Autodesk Inventor part; units mm, degrees
ref_plane "YZ Plane" through (0, 0, 0) normal (1, 0, 0) x (0, 1, 0)
ref_plane "XZ Plane" through (0, 0, 0) normal (0, 1, 0) x (-1, 0, 0)
ref_plane "XY Plane" through (0, 0, 0) normal (0, 0, 1) x (1, 0, 0)
sketch "Boceto1" plane through (0, 0, 0) normal (0, 1, 0) x (-1, 0, 0)
  line L0 (-50, 50) -> (50, 50)
  line L1 (50, 50) -> (50, -50)
  line L2 (50, -50) -> (-50, -50)
  line L3 (-50, -50) -> (-50, 50)
  line L4 (-50, 50) -> (50, -50) construction
  line L5 (50, 50) -> (-50, -50) construction
  point P0 (0, 0)
  dimension "d0" = 100
  dimension "d1" = 100
extrude "Extrusión1" add sketch "Boceto1" along normal blind 10
sketch "Boceto3" plane through (0, 10, 0) normal (0, 1, 0) x (1, 0, 0)
  point P0 (0, 0)
sketch "Boceto4" plane through (0, 10, 0) normal (0, 1, 0) x (1, 0, 0)
  circle A0 centre (0, 0) radius 45
  dimension "d5" = 90
extrude "Extrusión2" add sketch "Boceto4" along normal blind 20.06
sketch "Boceto5" plane through (0, 30.06, 0) normal (0, 1, 0) x (1, 0, 0)
  circle A0 centre (0, 0) radius 50
extrude "Extrusión3" add sketch "Boceto5" along normal blind 10
sketch "Boceto6" plane through (0, 40.06, 0) normal (0, 1, 0) x (1, 0, 0)
  circle A0 centre (0, 0) radius 15.325
  dimension "d10" = 30.65
hole "Agujero1" at (0, 40.06, 0) direction (0, -1, 0) diameter 30.65 end through all
properties part number "base de las bobinas"
Geometry: final body of the model. Coordinates: model frame, mm. A direction names the side the tool comes from. Coordinates: 2 decimals unless noted, no trailing zeros. Loops run counter-clockwise (first coordinate to the right, second up) from the corner with the lowest first, then second, coordinate; pieces in that order, holes last. Notation, with made-up numbers: M 31,9 L 35,9 A35 cw 35,42 Z; hole C 38,-22 d5. An arc over 180 degrees is marked long. One line per item, written item: value. Start each with the question number.
1) Cut plane A-A (z = 0). Return loops of the section in (x, y) (3 decimals), then the cut area to 3 significant figures.
2) Cut plane C-C (y = 35.5). Return loops of the section in (x, z) (3 decimals), then the cut area to 3 significant figures.
3) Material intervals for L1, parallel to Z at x = 0, y = 11 (3 decimals); L2, parallel to Y at x = 46.5, z = -11, sorted ascending. Write a range as from..to.
4) Pin query (flat end, axial travel): P1, Ø1.5, axis at x = -20, y = 35, coming from the +Z side; P2, Ø12, axis at y = 15, z = -18, coming from the -X side; P3, Ø6, axis at x = -37.5, y = 33.5, coming from the -Z side; P4, Ø4, axis at y = 22.5, z = 10.5, coming from the +X side. Return the tip coordinate at first contact, or that it passes through.
5) Draft query along Y for faces 1 (the flat face through (12, 0, 12)), 2 (the cylindrical face through (-12.92, 19.75, 8.24)), 3 (the cylindrical face through (20.765, 19.89, -39.923)). Return one class per face: released by +Y, released by -Y, zero draft, split by the parting line, or undercut.
6) Cut plane D-D (x = -22.5). Return loops of the section in (y, z), then the cut area to 3 significant figures.
7) Cut plane B-B (x = 0). Return loops of the section in (y, z) (3 decimals), then the cut area to 3 significant figures.
8) Reachability of faces 4 (the flat face through (50, 5, -1)), 5 (the flat face through (45, 10, 12)), 6 (the cylindrical face through (47.69, 34.99, 15.02)) from +Z, -Z, +X, -X, +Y, -Y: full face, straight path, thin tool, end or side. Return the list, or none.
Evaluation:
1. outline: M -50,0 L -15.325,0 L -15.325,40.06 L -50,40.06 L -50,30.06 L -45,30.06 L -45,10 L -50,10 Z; M 15.325,0 L 50,0 L 50,10 L 45,10 L 45,30.06 L 50,30.06 L 50,40.06 L 15.325,40.06 Z
1. area: 2,580 mm^2
2. outline: C 0,0 d100; hole C 0,0 d30.65
2. area: 7,120 mm^2
3. L1: -45..-15.325, 15.325..45
3. L2: 0..10, 30.06..40.06
4. P1: z = 46.15
4. P2: x = -50
4. P3: z = -36.19
4. P4: x = 44.19
5. face 1: released by -Y
5. face 2: zero draft
5. face 3: undercut
6. outline: M 0,-50 L 10,-50 L 10,-38.97 L 30.06,-38.97 L 30.06,-44.65 L 40.06,-44.65 L 40.06,44.65 L 30.06,44.65 L 30.06,38.97 L 10,38.97 L 10,50 L 0,50 Z
6. area: 3,460 mm^2
7. outline: M 0,-50 L 10,-50 L 10,-45 L 30.06,-45 L 30.06,-50 L 40.06,-50 L 40.06,-15.325 L 0,-15.325 Z; M 0,15.325 L 40.06,15.325 L 40.06,50 L 30.06,50 L 30.06,45 L 10,45 L 10,50 L 0,50 Z
7. area: 2,580 mm^2
8. face 4: +Z, -Z, +X, +Y, -Y
8. face 5: none
8. face 6: +Y
